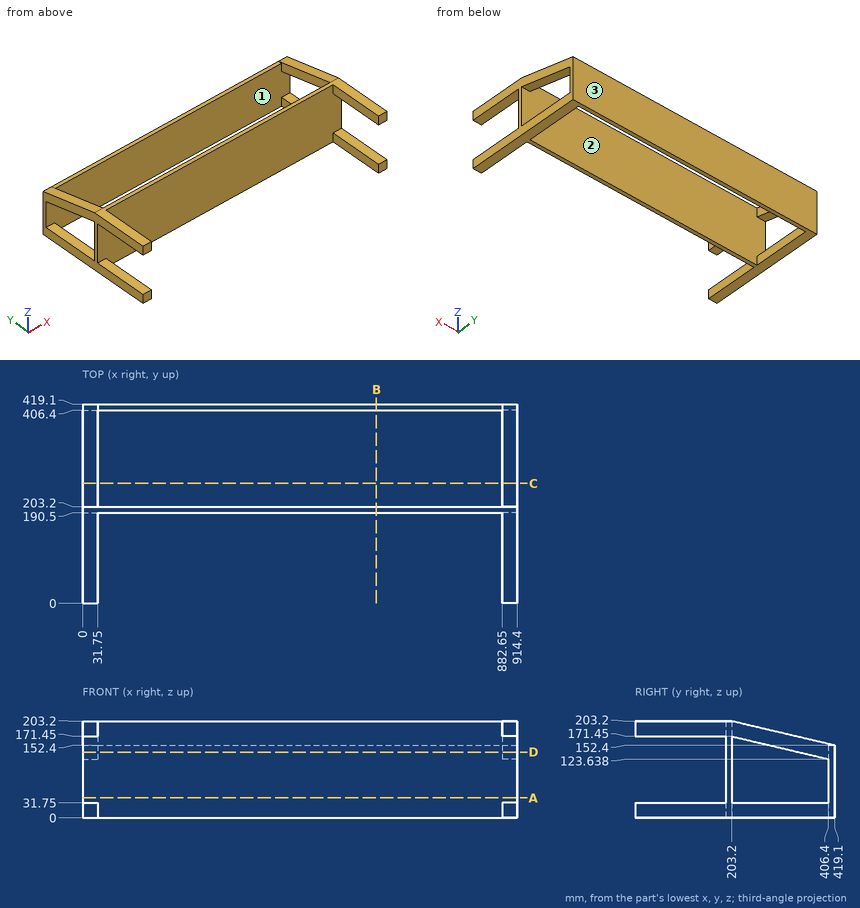
Source: three-view drawing plus pictorial views. Frame: mm from the lowest corner of the part. Round coordinates to 2 decimals unless told otherwise and drop trailing zeros. Write each loop counter-clockwise with the first axis right and the second up, starting at its lowest first coordinate (ties: lowest second). Pieces come first, ordered by that corner, then holes. Notation, with made-up numbers: M -19,53 L -5,53 A11 ccw -5,70 Z; hole C 34.5,-15.5 d11. An arc over 180 degrees is marked long. One line per item, written item: value. Start each with the question number.
Item 1: Mould query, pull axis Y, two halves, no side actions, for the marked faces 1, 2 and 3. Classes: pulls with the +Y half, pulls with the -Y half, needs draft (parallel to the pull), parting line crosses it, or undercut.
Item 2: Section query D-D (z = 138.5). Return the cut outline in (x, y).
Item 3: Section query C-C (y = 252). Return the cut outline in (x, z), plus the area to 3 significant figures.
Item 4: Ray query, L1, parallel to X at y = 223.5, z = 172.5; L2, parallel to Y at x = 156.5, z = 50.5; L3, parallel to Y at x = 606.5, z = 166.5. Return the intervals inside material, ascending. Write a range as from..to.
Item 5: Section query B-B (x = 618). Return the cut outline in (y, z), plus the area to 3 significant figures.
Item 6: Section query A-A (z = 42). Return the cut outline in (x, y).
Item 7: Pin query (flat end, axial travel): pin 1 (10 mm diameter, centred on x = 434.5, z = 115.5, fed in from -Y); pin 2 (14 mm diameter, centred on x = 558, y = 413, fed in from +Z); pin 3 (16 mm diameter, centred on x = 902.5, y = 289.5, fed in from +Z). Return the tip coordinate at first contact, or that it passes through.
Result set:
1. face 1: undercut
1. face 2: undercut
1. face 3: pulls with the +Y half
2. outline: M 0,190.5 L 914.4,190.5 L 914.4,203.2 L 0,203.2 Z; M 0,343.24 L 31.75,343.24 L 31.75,406.4 L 882.65,406.4 L 882.65,343.24 L 914.4,343.24 L 914.4,419.1 L 0,419.1 Z
3. outline: M 0,0 L 31.75,0 L 31.75,31.75 L 0,31.75 Z; M 0,159.97 L 31.75,159.97 L 31.75,191.72 L 0,191.72 Z; M 882.65,0 L 914.4,0 L 914.4,31.75 L 882.65,31.75 Z; M 882.65,159.97 L 914.4,159.97 L 914.4,191.72 L 882.65,191.72 Z
3. area: 4,030 mm²
4. L1: x = 0..31.75, 882.65..914.4
4. L2: y = 190.5..203.2, 406.4..419.1
4. L3: y = 190.5..203.2
5. outline: M 190.5,0 L 203.2,0 L 203.2,203.2 L 190.5,203.2 Z; M 406.4,0 L 419.1,0 L 419.1,152.4 L 406.4,152.4 Z
5. area: 4,520 mm²
6. outline: M 0,190.5 L 914.4,190.5 L 914.4,203.2 L 0,203.2 Z; M 0,406.4 L 914.4,406.4 L 914.4,419.1 L 0,419.1 Z
7. pin 1: stops at y = 190.5
7. pin 2: stops at z = 152.4
7. pin 3: stops at z = 184.78
